Here's the drawing with two shaded views (mm, measured from the low corner). I have some questions. A direction names the side the tool comes from. Coordinates: 2 decimals unless noted, no trailing zeros. Write each loop counter-clockwise with the first axis right and the second up, starting at its lowest first coordinate (ties: lowest second). Pieces come first, ordered by that corner, then holes. Notation, with made-up numbers: (35, 26) - (68, 26) arc R21 cw to (68, 62) - close; hole circle Ø4 at (-22, 62). An arc over 180 degrees is marked (long way). Answer in a Markdown table with one row per item. Add a question column.
Item 1: Which directions (+Z, -Z, +X, -X, +Y, -Y) give clear straight access to the entire face, cutting with the end or side of a thin tool? Please do the marked faces 1, 2, 3, 4 and 5.
Item 2: Imagine slicing it at D-D (z = 4). Please give me the cut outline in (x, y), plus the area to 3 significant figures.
Item 3: Imagine slicing it at C-C (x = 5.5). Please give me the cut outline in (y, z).
Item 4: If I drill on probe 1 along Z at (x, y) = (5, 6.5); probe 2 along Z at (x, y) = (7.5, 1.75); probe 3 along Y at (x, z) = (6.25, 7.75), over which ranges is the centre line in solid material (lowest first)? Write a range as from..to.
Item 5: I'm going to push flat-ended pins straight in: pin 1 (4 mm diameter, centred on x = 4, y = 2, fed in from +Z); pin 2 (4.5 mm diameter, centred on x = 4.5, z = 5, fed in from +Y); pin 3 (1.9 mm diameter, centred on x = 4, z = 6, fed in from -Y); pin 4 (0.8 mm diameter, centred on x = 4.5, y = 2.5, fed in from +Z). Where does each tip first touch, or does it pass through?
Item 6: Imagine slicing it at A-A (y = 6.5). Please give me the cut outline in (x, z).
Item 7: We'd pull the mould along X, two halves only. Please class the marked faces 6, 7 and 8: +X half, -X half, draft (parallel to the pull), parting line (faces both ways), or undercut.
Item 8: Imagine slicing it at B-B (z = 9). Please give me the cut outline in (x, y).
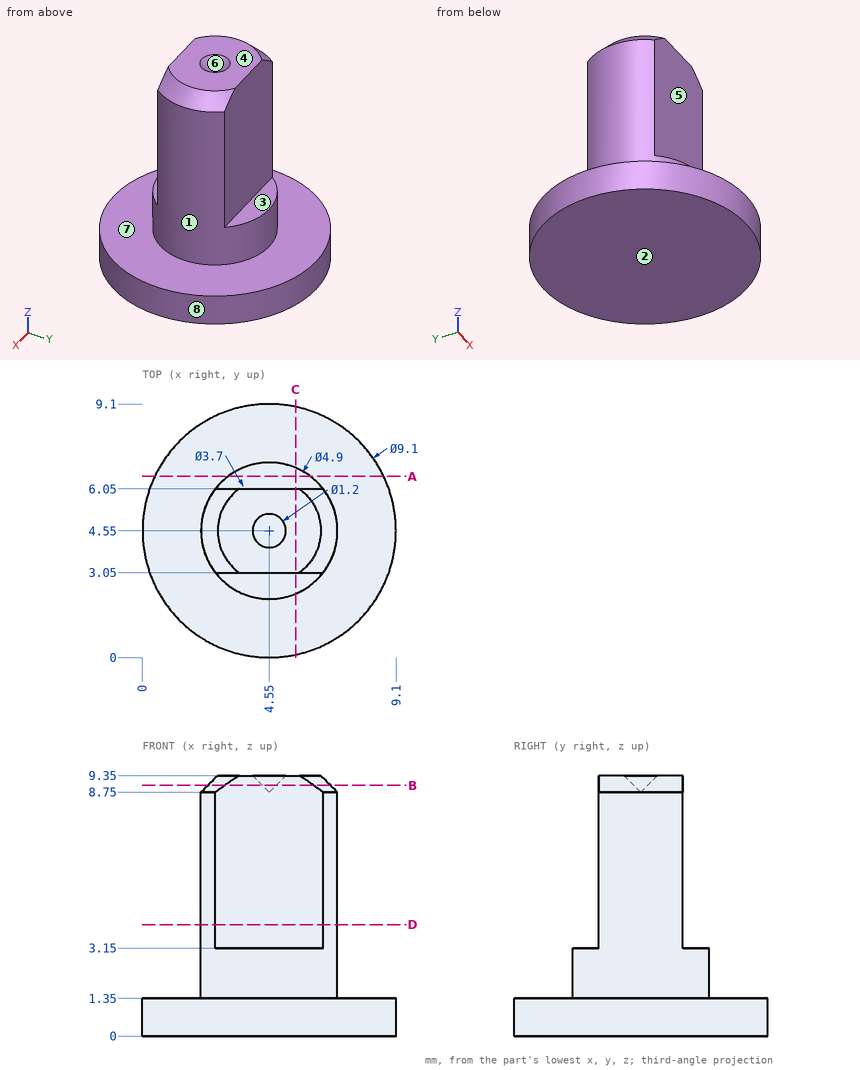
Here are the results:
| question | item | result |
|---|---|---|
| 1 | face 1 | +Z |
| 1 | face 2 | -Z, +X, -X, +Y, -Y |
| 1 | face 3 | +Z, +X, -X, +Y |
| 1 | face 4 | +Z, +X, -X, +Y, -Y |
| 1 | face 5 | +Z, +X, -X, -Y |
| 2 | outline | (2.61, 3.05) - (6.49, 3.05) arc R2.45 ccw to (6.49, 6.05) - (2.61, 6.05) arc R2.45 ccw to start |
| 2 | area | 13.7 mm2 |
| 3 | outline | (0.1, 0) - (9, 0) - (9, 1.35) - (6.81, 1.35) - (6.81, 3.15) - (6.05, 3.15) - (6.05, 9.35) - (3.05, 9.35) - (3.05, 3.15) - (2.29, 3.15) - (2.29, 1.35) - (0.1, 1.35) - close |
| 4 | probe 1 | z = 0..3.15 |
| 4 | probe 2 | z = 0..1.35 |
| 4 | probe 3 | y = 3.05..6.05 |
| 5 | pin 1 | stops at z = 9.35 |
| 5 | pin 2 | stops at y = 7 |
| 5 | pin 3 | stops at y = 3.05 |
| 5 | pin 4 | stops at z = 3.15 |
| 6 | outline | (0.44, 0) - (8.66, 0) - (8.66, 1.35) - (6.03, 1.35) - (6.03, 3.15) - (3.07, 3.15) - (3.07, 1.35) - (0.44, 1.35) - close |
| 7 | face 6 | undercut |
| 7 | face 7 | draft |
| 7 | face 8 | parting line |
| 8 | outline | (2.94, 3.05) - (6.16, 3.05) arc R2.2 ccw to (6.16, 6.05) - (2.94, 6.05) arc R2.2 ccw to start; hole circle Ø0.5 at (4.55, 4.55) |
